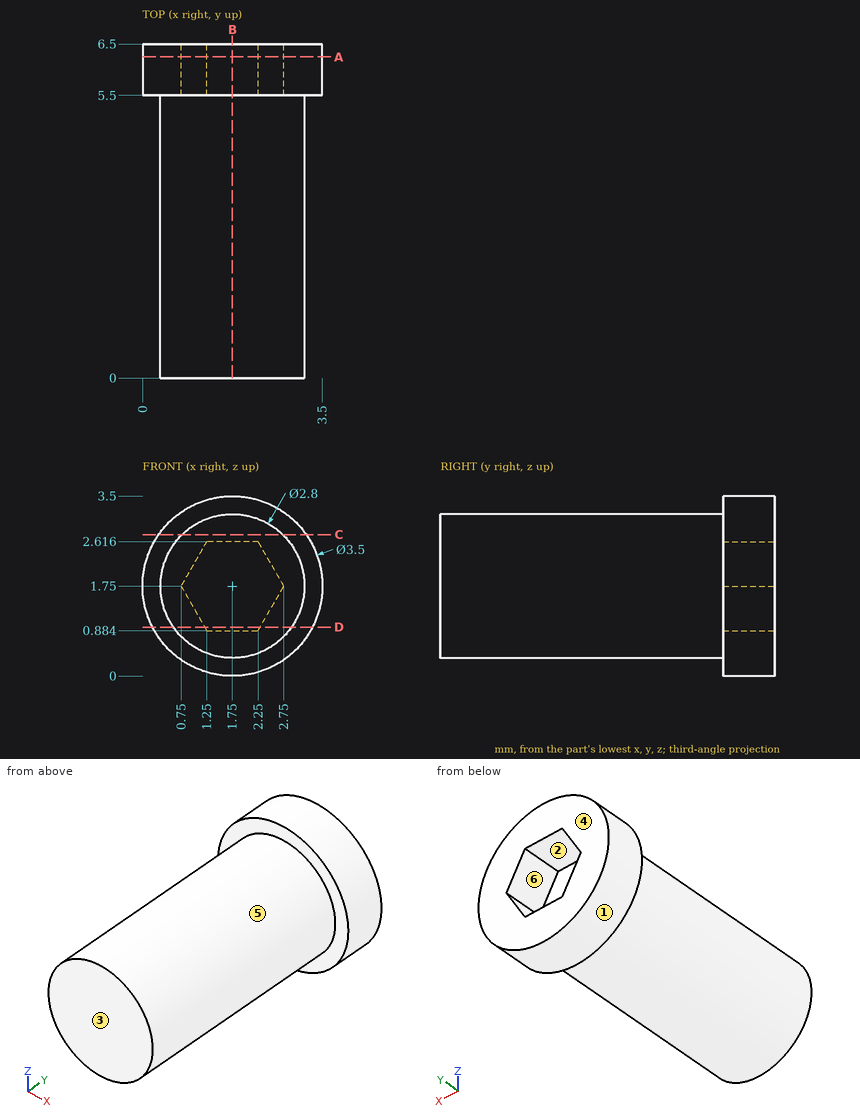
Design review of the part shown in the three views and the two pictorial views. Dimensions are in mm from the part's minimum x, y and z. A direction names the side the tool comes from. Coordinates: 2 decimals unless noted, no trailing zeros. Write each loop counter-clockwise with the first axis right and the second up, starting at its lowest first coordinate (ties: lowest second). Pieces come first, ordered by that corner, then holes.
1) Clearance check with flat-ended pins moving along their axes: pin 1 Ø0.5 at (x, z) = (2, 1.5) entering from +Y; pin 2 Ø1.5 at (x, y) = (2, 3) entering from +Z. State where each tip first meets the part, or that it passes through.
2) We need section C-C on z = 2.75. State the section outline as (x, y) points.
3) Machinability: for the marked faces 4, 5 and 6, which of the approach directions +Z, -Z, +X, -X, +Y, -Y give a long, thin tool a straight path to every point of the face, cutting with its end or side? Answer none if there is none.
4) The part is to be moulded in two halves that separate along X. For the marked faces 1, 2 and 3, say which applies: pulls with the +X half, pulls with the -X half, needs draft (parallel to the pull), parting line crosses it, or undercut.
5) We need section D-D on z = 0.95. State the section outline as (x, y) points, then the cut area to 3 significant figures.
6) We need section B-B on x = 1.75. State the section outline as (y, z) points.
7) We need section A-A on y = 6.25. State the section outline as (x, z) points, then the cut area to 3 significant figures.
8) To check wall thickness, follow probe 1 along Y at (x, z) = (2.35, 1.2); probe 2 along Y at (x, z) = (2.85, 0.75); probe 3 along Z at (x, y) = (1.7, 0.75). State the ranges of each line that lie inside material, in increasing order.
Answer list:
1. pin 1: stops at y = 5.5
1. pin 2: stops at z = 3.15
2. outline: (0.31, 5.5) - (0.77, 5.5) - (0.77, 0) - (2.73, 0) - (2.73, 5.5) - (3.19, 5.5) - (3.19, 6.5) - (0.31, 6.5) - close
3. face 4: +Z, -Z, +X, -X, +Y
3. face 5: -Y
3. face 6: +Y
4. face 1: parting line crosses it
4. face 2: undercut
4. face 3: needs draft
5. outline: (0.19, 5.5) - (0.6, 5.5) - (0.6, 0) - (2.9, 0) - (2.9, 5.5) - (3.31, 5.5) - (3.31, 6.5) - (2.29, 6.5) - (2.29, 5.5) - (1.21, 5.5) - (1.21, 6.5) - (0.19, 6.5) - close
5. area: 14.7 mm2
6. outline: (0, 0.35) - (5.5, 0.35) - (5.5, 0) - (6.5, 0) - (6.5, 0.88) - (5.5, 0.88) - (5.5, 2.62) - (6.5, 2.62) - (6.5, 3.5) - (5.5, 3.5) - (5.5, 3.15) - (0, 3.15) - close
7. outline: circle Ø3.5 at (1.75, 1.75); hole (0.75, 1.75) - (1.25, 0.88) - (2.25, 0.88) - (2.75, 1.75) - (2.25, 2.62) - (1.25, 2.62) - close
7. area: 7.02 mm2
8. probe 1: y = 0 to 5.5
8. probe 2: y = 5.5 to 6.5
8. probe 3: z = 0.35 to 3.15
